```python
from build123d import *

# Parameters (mm, degrees)
BOSS_EXTRUDE1_DEPTH = 31.75
SKETCH2_R           = 4.7625
SKETCH2_R_2         = 7.9375
CUT_EXTRUDE1_DEPTH  = 9.525
SKETCH2_4_R         = 4.7625
CUT_EXTRUDE2_DEPTH  = 42.275
CUT_EXTRUDE3_DEPTH  = 48.81496526
CHAMFER1_SIZE       = 6.35


with BuildPart() as part:
    # Sketch1 → Boss-Extrude1 (new body, symmetric)
    with BuildSketch(Plane(origin=(0, 0, 0), x_dir=(0, 0, -1), z_dir=(1, 0, 0))):
        Polygon((20.6375, 76.2), (20.6375, 0), (-20.6375, 0), (-20.6375, 57.15), (-1.5875, 57.15), (-1.5875, 76.2), align=None)
    extrude(amount=BOSS_EXTRUDE1_DEPTH, both=True)

    # Sketch2 → Cut-Extrude1 (cut)
    with BuildSketch(Plane.XY.offset(20.6375)):
        with Locations((-14.2875, 17.4625)):
            Circle(SKETCH2_R)
        with Locations((14.2875, 17.4625)):
            Circle(SKETCH2_R)
        with Locations((14.2875, 17.4625)):
            Circle(SKETCH2_R_2)
        with Locations((14.2875, 17.4625)):
            Circle(SKETCH2_R, mode=Mode.SUBTRACT)
        with Locations((-14.2875, 17.4625)):
            Circle(SKETCH2_R_2)
        with Locations((-14.2875, 17.4625)):
            Circle(SKETCH2_R, mode=Mode.SUBTRACT)
    extrude(amount=-CUT_EXTRUDE1_DEPTH, mode=Mode.SUBTRACT)

    # Sketch2_4 → Cut-Extrude2 (cut, through all)
    with BuildSketch(Plane.XY.offset(20.6375)):
        with Locations((-14.2875, 17.4625)):
            Circle(SKETCH2_4_R)
        with Locations((14.2875, 17.4625)):
            Circle(SKETCH2_4_R)
    extrude(amount=-CUT_EXTRUDE2_DEPTH, mode=Mode.SUBTRACT)

    # Sketch3 → Cut-Extrude3 (cut, through all, along a direction that is not the sketch's normal)
    with BuildSketch(Plane.XY.offset(20.6375)):
        Polygon((-39.6875, 76.2), (-3.175, 39.6875), (-3.175, 34.925), (3.175, 34.925), (3.175, 39.6875), (39.6875, 76.2), align=None)
    extrude(amount=-CUT_EXTRUDE3_DEPTH, dir=(0, -0.5, 0.866025404), mode=Mode.SUBTRACT)

    # Chamfer1
    chamfer1_edges = [part.edges().sort_by_distance(p)[0] for p in [
        (31.75, 28.575, 20.6375),
        (-31.75, 28.575, 20.6375),
    ]]
    chamfer(chamfer1_edges, length=CHAMFER1_SIZE)


solid = part.part
```
The model under review builds one solid part; all positions refer to its coordinate system, in mm. A direction names the side the tool comes from. Round coordinates to 2 decimals unless told otherwise and drop trailing zeros. Order: outer loops, then holes, each group sorted by start corner. A loop starts at its lowest first (then second) coordinate and runs counter-clockwise, first axis right, second up. Notation, with made-up numbers: (38, 23) -> (81, 23) arc R17 cw to (81, 52) -> close; hole circle Ø2 at (72.25, 67.5). An arc over 180 degrees is marked (long way). One line per item, written item: value. Start each with the question number.
Q1. Machinability: for faces 4 (the face through (26, 76.2, -12)), 5 (the face through (-14, 12, 11.112)), 6 (the face through (-23, 57.15, 9)), 7 (the face through (-3.175, 49, -1)), which of the approach directions +Z, -Z, +X, -X, +Y, -Y give a long, thin tool a straight path to every point of the face, cutting with its end or side? Answer none if there is none.
Q2. Wall thickness on line 1 (X direction, y = 18, z = -15.5); line 2 (Y direction, x = -24, z = 5); line 3 (Y direction, x = -15.5, z = -4.5): over which ranges is each line inside the solid? List them lowest first.
Q3. Take a section at B-B (z = -7). Count the separate pieces of the cut face and the enclosed holes in it, and give its area (3 significant figures).
Q4. Mouldability with a two-part tool opening along X and no side actions: class faces 1 (the face through (28.53, 28.17, 17.51)), 2 (the face through (-9.745, 18.893, -4.54)), 3 (the face through (0, 28, 20.638)) as released by +X, released by -X, zero draft, split by the parting line, or undercut.
Q5. Clearance check with flat-ended pins moving along their axes: pin 1 Ø5.5 at (x, z) = (-15.5, 15.5) entering from +Y; pin 2 Ø5.5 at (x, y) = (18, 68) entering from +Z; pin 3 Ø21 at (x, z) = (16, 13.5) entering from +Y. State where each tip first meets the part, or that it passes through.
Q6. Take a section at A-A (x = -11). Write out the cut boundary in (y, z), and give its area (3 significant figures).
Reported:
1. face 4: +Z, -Z, +X, -X, +Y
1. face 5: +Z
1. face 6: +Z, +X, -X, +Y
1. face 7: +Z, +Y
2. line 1: x = -31.75 to -19.02, -9.56 to 9.56, 19.02 to 31.75
2. line 2: y = 0 to 57.15
2. line 3: y = 0 to 12.86, 22.07 to 66.53
3. separate pieces: 1
3. enclosed holes: 2
3. area: 4,110 mm2
4. face 1: released by +X
4. face 2: undercut
4. face 3: zero draft
5. pin 1: stops at y = 57.15
5. pin 2: stops at z = 1.59
5. pin 3: stops at y = 57.15
6. outline: (0, -20.64) -> (14.02, -20.64) -> (14.02, 11.11) -> (10.24, 11.11) -> (10.24, 20.64) -> (0, 20.64) -> close; (20.91, -20.64) -> (71.34, -20.64) -> (58.51, 1.59) -> (57.15, 1.59) -> (57.15, 3.94) -> (47.51, 20.64) -> (24.69, 20.64) -> (24.69, 11.11) -> (20.91, 11.11) -> close
6. area: 2,090 mm2
